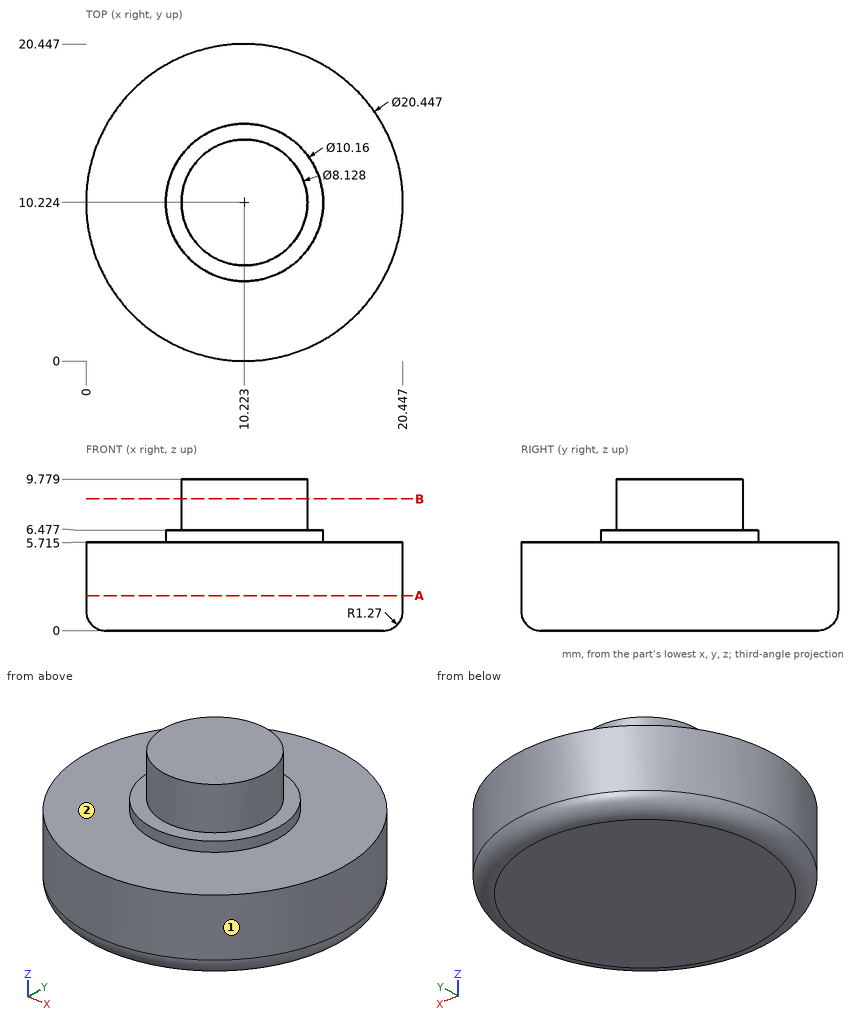
Geometry check sheet. Reference: drawing and pictorial views, mm from the part's lowest x, y, z. A direction names the side the tool comes from. Coordinates: 2 decimals unless noted, no trailing zeros. Loops run counter-clockwise (first coordinate to the right, second up) from the corner with the lowest first, then second, coordinate; pieces in that order, holes last.
1) Material ranges on probe 1 along Z at (x, y) = (7.5, 15.75) (1 decimal); probe 2 along Y at (x, z) = (11.5, 1.25); probe 3 along X at (y, z) = (18.5, 5.5) (1 decimal), recorded low to high.
2) Gauge pin test, flat end, axial feed: pin 1 (1 mm diameter, centred on y = 14, z = 3.5, fed in from +X). Record the tip position at first contact, or that the pin passes through.
3) Access from +Z, -Z, +X, -X, +Y, -Y to the whole of each face (thin tool, end or side, straight path). Record for the marked faces 1 and 2.
4) Sectioned sample at B-B (z = 8.5). Record the boundary of the cut face in (x, y) (1 decimal).
5) Sectioned sample at A-A (z = 2.25). Record the boundary of the cut face in (x, y).
Check sheet entries:
1. probe 1: z = 0 to 5.7
1. probe 2: y = 0.08 to 20.37
1. probe 3: x = 4.2 to 16.2
2. pin 1: stops at x = 19.91
3. face 1: +Z, -Z
3. face 2: +Z
4. outline: circle Ø8.1 at (10.2, 10.2)
5. outline: circle Ø20.45 at (10.22, 10.22)
